Verification items for the finished model (mm, model axes). Face numbers are marked on the shaded views. A direction names the side the tool comes from. Round coordinates to 2 decimals unless told otherwise and drop trailing zeros. Order: outer loops, then holes, each group sorted by start corner. A loop starts at its lowest first (then second) coordinate and runs counter-clockwise, first axis right, second up. Notation, with made-up numbers: M 69,8 L 85,8 A20 ccw 85,34 Z; hole C 5.5,36.25 d9. An arc over 180 degrees is marked long. Use one line per item in the form item = value. Start each with the question number.
Item 1: Go/stop test with flat-tipped pins: pin 1 Ø6 at (x, y) = (-20, 7.5) entering from +Z; pin 2 Ø12.5 at (x, z) = (-2.5, 27) entering from -Y; pin 3 Ø21 at (x, z) = (17.5, 25.5) entering from +Y. Record where each tip stops, or that it passes through.
Item 2: Cross-section at C-C on y = -10. Enter the section's corners in (x, z), then the cut area to 3 significant figures.
Item 3: Thickness scan on probe 1 along Z at (x, y) = (8, 18.5); probe 2 along X at (y, z) = (7.5, 36); probe 3 along Y at (x, z) = (-0.5, 26.5). Record the ranges inside material, lowest first. Write a range as [from, to].
Item 4: Cross-section at B-B on z = 36. Enter the section's corners in (x, y), then the cut area to 3 significant figures.
Item 5: Tool access check on the marked faces 1, 2, 3 and 4. Record the directions out of +Z, -Z, +X, -X, +Y, -Y that give a thin tool (end or side, any length) a straight path to the whole face; none if there is none.
Item 6: Cross-section at A-A on x = 19.5. Enter the section's corners in (y, z).
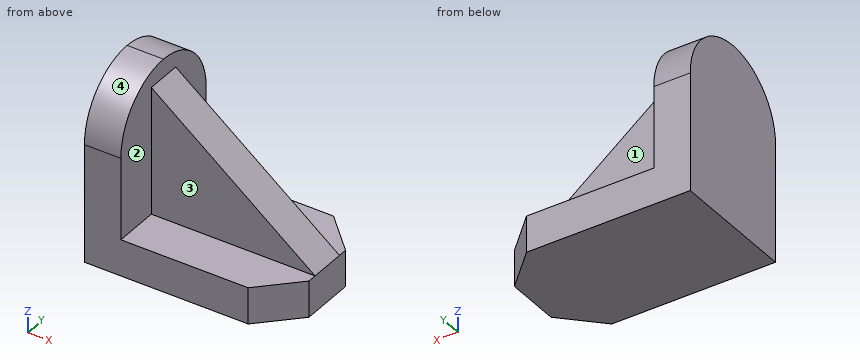
Autodesk Fusion 360 part; units mm, degrees
sketch "the horizontal part sketch" plane through (0, 0, 0) normal (0, 0, 1) x (1, 0, 0)
  line L0 (-33, 21) -> (33, 21)
  line L1 (33, 21) -> (33, -21)
  line L2 (33, -21) -> (-33, -21)
  line L3 (-33, -21) -> (-33, 21)
  line L4 (-33, 21) -> (33, -21) construction
  line L5 (33, 21) -> (-33, -21) construction
  dimension "d1" = 66
  dimension "d2" = 42
extrude "Extrude1" add sketch "the horizontal part sketch" along normal blind 12 makes body 1
sketch "the vertical part sketch" plane through (0, 0, 12) normal (0, 0, 1) x (-1, 0, 0)
  line L0 (33, 21) -> (-33, 21)
  line L1 (-33, 21) -> (-33, -21)
  line L2 (-33, -21) -> (33, -21)
  line L3 (33, -21) -> (33, 21)
  line L4 (33, -21) -> (21, -21)
  line L5 (21, -21) -> (21, 21)
  line L6 (21, 21) -> (33, 21)
  line L7 (33, 21) -> (33, -21)
  dimension "d5" = 12
extrude "Extrude2" add sketch "the vertical part sketch" along normal blind 48 contours L0 L2 L3 L4 L5 L6 L7 bodies 1
fillet "Fillet1" radius 21 1 edges at (-27, -21, 60) on bodies 1
fillet "Fillet2" radius 21 1 edges at (-27, 21, 60) on bodies 1
chamfer "Chamfer1" distance 12 angle 45 1 edges at (33, 21, 6) on bodies 1
chamfer "Chamfer2" distance 12 angle 45 1 edges at (33, -21, 6) on bodies 1
sketch "triangle sketch" plane through (0, 0, 0) normal (0, 1, 0) x (1, 0, 0)
  line L0 (-21, -54) -> (-21, -12)
  line L1 (-21, -12) -> (33, -12)
  line L2 (33, -12) -> (-21, -54)
  dimension "d14" = 42
  dimension "d15" = 54
extrude "Extrude3" add sketch "triangle sketch" along normal mid plane 12 bodies 1
copy_body "Body->Comp1" bodies 1 removing the originals makes body 2 in component "object A1"
component "object A1" placed x (1, 0, 0) y (0, 1, 0) z (0, 0, 1) at (0, 0, 0)
equation "d6 = 60 mm - 12 mm"
equation "d15 = 66 mm - 12 mm"
Output values:
q1.pin_1 = 59.47
q1.pin_2 = -6
q1.pin_3 = 6
q2.outline = M -33,0 L 32,0 L 32,12 L -21,12 L -21,57.47 L -33,57.47 Z
q2.area = 1,330 mm2
q3.probe_1 = [0, 12]
q3.probe_2 = [-33, -21]
q3.probe_3 = [-6, 6]
q4.outline = M -33,-21 L -21,-21 L -21,-6 L 2.14,-6 L 2.14,6 L -21,6 L -21,21 L -33,21 Z
q4.area = 782 mm2
q5.face_1 = +Z, +X, +Y
q5.face_2 = +Z, +X
q5.face_3 = +Z, +X, -Y
q5.face_4 = +Z, +X, -X, -Y
q6.outline = M -21,0 L 21,0 L 21,12 L 6,12 L 6,22.5 L -6,22.5 L -6,12 L -21,12 Z
